Autodesk Inventor part; units mm, degrees
ref_plane "YZ Plane" through (0, 0, 0) normal (1, 0, 0) x (0, 1, 0)
ref_plane "XZ Plane" through (0, 0, 0) normal (0, 1, 0) x (-1, 0, 0)
ref_plane "XY Plane" through (0, 0, 0) normal (0, 0, 1) x (1, 0, 0)
sketch "スケッチ1" plane through (0, 0, 0) normal (1, 0, 0) x (0, 1, 0)
  line L0 (-15, -27) -> (-15, 27)
  line L1 (-15, 27) -> (15, 27)
  line L2 (15, 27) -> (15, -27)
  line L3 (15, -27) -> (-15, -27)
  line L4 (-15, -27) -> (15, 27) construction
  line L5 (-15, 27) -> (15, -27) construction
  point P0 (0, 0)
  dimension "d0" = 30
  dimension "d1" = 54
extrude "プレート1" add sketch "スケッチ1" along normal blind 1.5
sketch "スケッチ2" plane through (1.5, -15, 27) normal (0, 0, 1) x (1, 0, 0)
  line L0 (0, 30) -> (0, 0)
  line L1 (0, 0) -> (48.5, 0)
  line L2 (48.5, 0) -> (48.5, 30)
  line L3 (48.5, 30) -> (0, 30)
edge flange "フランジ1" height 50 angle 90 thickness 1.5 bend radius 1.5 thickness toward (0, 0, 1) relief tear relief width 1.5 relief depth 0.75 corner gap 1.5 corner form 0 edges at (1.5, 0, 27) (1.5, 0, -27) wall of the first edge with corners at (1.5, 15, 27) (1.5, -15, 27) (50, -15, 27) (50, 15, 27)
bend "曲げ1"
corner "コーナー1"
sketch "スケッチ3" plane through (50, 15, 28.5) normal (1, 0, 0) x (0, 1, 0)
  line L0 (-30, 0) -> (0, 0)
  line L1 (0, 0) -> (0, 13.5)
  line L2 (0, 13.5) -> (-30, 13.5)
  line L3 (-30, 13.5) -> (-30, 0)
edge flange "フランジ2" height 15 angle 90 thickness 1.5 bend radius 1.5 thickness toward (1, 0, 0) relief tear relief width 1.5 relief depth 0.75 corner gap 1.5 corner form 0 edges at (50, 0, 28.5) (50, 0, -28.5) wall of the first edge with corners at (50, -15, 28.5) (50, 15, 28.5) (50, 15, 42) (50, -15, 42)
bend "曲げ2"
corner "コーナー2"
sketch "スケッチ4" plane through (0, 0, 0) normal (-1, 0, 0) x (0, 0, 1)
  circle A0 centre (0, 0) radius 5
  circle A1 centre (10, 0) radius 1.35
  circle A2 centre (-5, 8.6603) radius 1.35
  circle A3 centre (-5, -8.6603) radius 1.35
  dimension "d23" = 10
  dimension "d24" = 2.7
  dimension "d25" = 0
  dimension "d26" = 10
  dimension "d29" = 360
extrude "押し出し1" cut sketch "スケッチ4" against normal blind 2
sketch "スケッチ6" plane through (50, -15, 42) normal (-1, 0, 0) x (0, 0, 1)
  circle A0 centre (-6, 24) radius 2
  line L0 (-12, 30) -> (0, 30)
  line L1 (0, 0) -> (0, 30)
  circle A1 centre (-6, 6) radius 2
  circle A2 centre (-78, 24) radius 2
  circle A3 centre (-78, 6) radius 2
  point P0 (-42, 15)
  dimension "d41" = 4
  dimension "d42" = 4
  dimension "d43" = 4
  dimension "d46" = 18
  dimension "d49" = 72
extrude "押し出し3" add sketch "スケッチ6" along normal blind 1.5
sketch "スケッチ7" plane through (48.5, 9, 36) normal (-1, 0, 0) x (0, 0, 1)
  circle A0 centre (0, 0) radius 2
  circle A1 centre (0, -18) radius 2
  circle A2 centre (-72, -18) radius 2
  circle A3 centre (-72, 0) radius 2
  circle A4 centre (0, 0) radius 2
  circle A5 centre (0, -18) radius 2
  circle A6 centre (-72, -18) radius 2
  point P0 (-36, -9)
hole "穴1" at (48.5, 9, 36) at (48.5, -9, 36) at (48.5, 9, -36) at (48.5, -9, -36) direction (1, 0, 0) diameter 2.459 depth 3
fillet "フィレット1" radius 5 4 edges at (50.75, 15, 42) (50.75, -15, 42) (50.75, 15, -42) (50.75, -15, -42)
sketch "スケッチ8" plane through (3, -15, -28.5) normal (0, 0, -1) x (-1, 0, 0)
  circle A0 centre (-29.65, 22) radius 1.6
  line L0 (-47, 25) -> (-47, 5)
  line L1 (-45.5, 30) -> (0, 30)
  circle A1 centre (-29.65, 8) radius 1.6
  point P0 (3, 15)
  dimension "d62" = 3.2
  dimension "d63" = 17.35
  dimension "d64" = 8
  dimension "d67" = 14
extrude "押し出し4" cut sketch "スケッチ8" against normal blind 10
equation "\"d59\" = Thickness"
equation "\"BendRadius\" = Thickness"
equation "\"BendReliefWidth\" = Thickness"
equation "\"BendReliefDepth\" = 0.5 * Thickness"
equation "\"CornerReliefSize\" = 4 * Thickness"
equation "\"MinimumRemnant\" = 2 * Thickness"
equation "\"TransitionRadius\" = BendRadius"
equation "\"JacobiRadiusSize\" = BendRadius"
equation "\"GapSize\" = Thickness"
properties part number "Old_hand_box2" material "アルミニウム 6061"
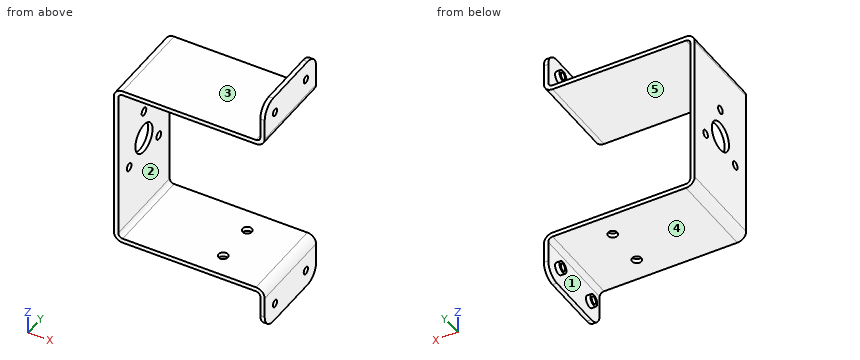
Here's how the part is built. I have some questions about the finished solid (model axes, mm). Face numbers are marked on the shaded views. A direction names the side the tool comes from. Round coordinates to 2 decimals unless told otherwise and drop trailing zeros. Order: outer loops, then holes, each group sorted by start corner. A loop starts at its lowest first (then second) coordinate and runs counter-clockwise, first axis right, second up. Notation, with made-up numbers: (57.25, 58) -> (64.25, 58) arc R15 ccw to (64.25, 72) -> close; hole circle Ø1 at (54, -9.5). An arc over 180 degrees is marked (long way). Return JSON: item names as keys, results as strings.
Q1. If we section it at B-B on x = 47: List the corners of the cut face in (y, z) for me, plus the area to 3 significant figures.
Filled sheet:
{"outline": "(-15, -28.5) -> (15, -28.5) -> (15, -27) -> (-15, -27) -> close; (-15, 27) -> (15, 27) -> (15, 28.5) -> (-15, 28.5) -> close", "area": "90.0 mm^2"}
Q2. I need wall thicknesses on line 1 along Y through (x, z) = (50.4, -36); line 2 along Y through (x, z) = (49.65, -36); line 3 along Z through (x, y) = (19, -0.5). Which ranges of each line are inside material? Lowest first, please. Write a range as from..to.
Filled sheet:
{"line 1": "y = -15..-10.23, -7.77..7.77, 10.23..15", "line 2": "y = -11..-10.23, -7.77..-7, 7..7.77, 10.23..11", "line 3": "z = -28.5..-27, 27..28.5"}
Q3. If we mould it in two halves opening along Y, with no side actions, what happens to the marked faces 1 and 2? For each: released by +Y, released by -Y, zero draft, split by the parting line, or undercut.
Filled sheet:
{"face 1": "undercut", "face 2": "zero draft"}
Q4. For pin 1 Ø3 at (x, y) = (32.65, 7) entering from +Z; pin 2 Ø15 at (y, z) = (-6.5, -9) entering from +X; pin 3 Ø5 at (y, z) = (-5.5, -22.5) entering from -X; pin 4 Ø2 at (y, z) = (8.66, -5) entering from -X, each with a flat end and sliding along its axis, tell me the tip position at first contact or that it passes through.
Filled sheet:
{"pin 1": "stops at z = 28.5", "pin 2": "stops at x = 1.5", "pin 3": "stops at x = 0", "pin 4": "passes through"}
Q5. If we section it at A-A on z = 0: List the corners of the cut face in (x, y) for me, plus the area to 3 significant figures.
Filled sheet:
{"outline": "(0, -15) -> (1.5, -15) -> (1.5, -5) -> (0, -5) -> close; (0, 5) -> (1.5, 5) -> (1.5, 15) -> (0, 15) -> close", "area": "30.0 mm^2"}
Q6. If we section it at C-C on z = 36: List the corners of the cut face in (x, y) for me.
Filled sheet:
{"outline": "(48.5, -11) -> (50, -11) -> (50, -15) -> (51.5, -15) -> (51.5, -10.23) -> (48.5, -10.23) -> close; (48.5, -7.77) -> (51.5, -7.77) -> (51.5, 7.77) -> (48.5, 7.77) -> (48.5, 7) -> (50, 7) -> (50, -7) -> (48.5, -7) -> close; (48.5, 10.23) -> (51.5, 10.23) -> (51.5, 15) -> (50, 15) -> (50, 11) -> (48.5, 11) -> close"}
Q7. If we section it at D-D on y = 0: List the corners of the cut face in (x, z) for me.
Filled sheet:
{"outline": "(0, -25.5) arc R3 ccw to (3, -28.5) -> (48.5, -28.5) arc R1.5 cw to (50, -30) -> (50, -42) -> (51.5, -42) -> (51.5, -30) arc R3 ccw to (48.5, -27) -> (3, -27) arc R1.5 cw to (1.5, -25.5) -> (1.5, -5) -> (0, -5) -> close; (0, 5) -> (1.5, 5) -> (1.5, 8.65) -> (0, 8.65) -> close; (0, 11.35) -> (1.5, 11.35) -> (1.5, 25.5) arc R1.5 cw to (3, 27) -> (48.5, 27) arc R3 ccw to (51.5, 30) -> (51.5, 42) -> (50, 42) -> (50, 30) arc R1.5 cw to (48.5, 28.5) -> (3, 28.5) arc R3 ccw to (0, 25.5) -> close"}
Q8. Which directions (+Z, -Z, +X, -X, +Y, -Y) give clear straight access to the entire face, cutting with the end or side of a thin tool? Please do the marked faces 3, 4 and 5.
Filled sheet:
{"face 3": "+Z, -X, +Y, -Y", "face 4": "-Z, -X, +Y, -Y", "face 5": "+X, +Y, -Y"}
